```python
from build123d import *

# Parameters (mm, degrees)
SKETCH1_W           = 304.8
SKETCH1_H           = 177.8
BOSS_EXTRUDE1_DEPTH = 228.6
SKETCH2_W           = 6.35
SKETCH2_H           = 29.137469297


with BuildPart() as part:
    # Sketch1 → Boss-Extrude1 (new body)
    with BuildSketch(Plane(origin=(0, 0, 0), x_dir=(1, 0, 0), z_dir=(0, 1, 0))):
        Rectangle(SKETCH1_W, SKETCH1_H)
    extrude(amount=BOSS_EXTRUDE1_DEPTH)

    # Sketch2 → Revolve1 (revolve)
    with BuildSketch(Plane(origin=(0, 152.4, 0), x_dir=(1, 0, 0), z_dir=(0, 1, 0))):
        with Locations((-155.575, 14.568734649)):
            Rectangle(SKETCH2_W, SKETCH2_H)
    revolve(axis=Axis((-152.4, 152.4, 0), (-1, 0, 0)))


solid = part.part
```
Design review of the part built by this model. Coordinates are the model's own, in mm. A direction names the side the tool comes from. Give positions to 0.01 mm unless a question says otherwise; leave off trailing zeros. Loops run counter-clockwise (first coordinate to the right, second up) from the corner with the lowest first, then second, coordinate; pieces in that order, holes last. Notation, with made-up numbers: M 55,45 L 66,45 A23 cw 66,65 Z; hole C 49,-0.75 d2. An arc over 180 degrees is marked long. Return JSON: item names as keys, results as strings. Group by question number.
Item 1: We need section A-A (z = 0). Give the boundary of the cut face in (x, y), and give its area (3 significant figures).
Item 2: For probe 1 along X at (y, z) = (192.5, 72), list the stretches that pass through material, from the lowest coordinate up.
Item 3: We need section C-C (z = 21). Give the boundary of the cut face in (x, y).
Item 4: We need section D-D (z = 52). Give the boundary of the cut face in (x, y), and give its area (3 significant figures).
Item 5: We need section B-B (y = 207.5). Give the boundary of the cut face in (x, z).
Item 6: Tool access review of faces 1 (the cylindrical face through (-155.53, 123.51, 3.79)), 2 (the flat face through (-2, 0, -1)): name each direction out of +Z, -Z, +X, -X, +Y, -Y from which nothing blocks a thin tool from reaching the whole face with its end or side.
Item 7: Insertion check: pin 1 Ø5 at (y, z) = (51.5, 44.5) entering from -X. The pin has a flat end and moves straight along its axis. Give the tip position at first contact, or say it passes through.
Output:
{
 "1": {"outline": "M -158.75,123.26 L -152.4,123.26 L -152.4,0 L 152.4,0 L 152.4,228.6 L -152.4,228.6 L -152.4,181.54 L -158.75,181.54 Z", "area": "70,000 mm^2"},
 "2": {"probe 1": "x = -152.4 to 152.4"},
 "3": {"outline": "M -158.75,132.2 L -152.4,132.2 L -152.4,0 L 152.4,0 L 152.4,228.6 L -152.4,228.6 L -152.4,172.6 L -158.75,172.6 Z"},
 "4": {"outline": "M -152.4,0 L 152.4,0 L 152.4,228.6 L -152.4,228.6 Z", "area": "69,700 mm^2"},
 "5": {"outline": "M -152.4,-88.9 L 152.4,-88.9 L 152.4,88.9 L -152.4,88.9 Z"},
 "6": {"face 1": "-X", "face 2": "+Z, -Z, +X, -X, -Y"},
 "7": {"pin 1": "stops at x = -152.4"}
}
